The model under review builds one solid part; all positions refer to its coordinate system, in mm. A direction names the side the tool comes from. Round coordinates to 2 decimals unless told otherwise and drop trailing zeros. Order: outer loops, then holes, each group sorted by start corner. A loop starts at its lowest first (then second) coordinate and runs counter-clockwise, first axis right, second up. Notation, with made-up numbers: M -29.5,25 L -12.5,25 A6 cw -12.5,29 Z; hole C 51,88 d11. An arc over 180 degrees is marked long. Answer as a JSON object with one key per item and string values. Group by question number.
1) For faces 1 (the flat face through (-63.5, 1, 0)), 2 (the flat face through (64.146, -12.31, -0.117)), 3 (the cylindrical face through (-41.186, 0.86, -3.874)), list the 3-axis set-ups (+Z, -Z, +X, -X, +Y, -Y) from which the entire face can be reached by the end or side of a thin tool; tool diameter is ignored.
2) Consider section A-A, the plane x = -38. Write out the cut boundary in (y, z), then the cut area to 3 significant figures.
3) The part is to be moulded in two halves that separate along X. For faces 4 (the conical face through (-55.451, 0.681, -3.065)), 5 (the cylindrical face through (-17.218, 0.647, -2.914)), 6 (the cylindrical face through (76.16, -7.92, 10.66)), say which applies: +X half, -X half, draft (parallel to the pull), parting line (faces both ways), or undercut.
4) To check wall thickness, follow line 1 (Z direction, x = -41, y = 0); line 2 (Z direction, x = -27, y = 0); line 3 (X direction, y = -11.5, z = 9.5). State the ranges of each line that lie inside material, in increasing order.
5) Consider section B-B, the plane x = -4. Write out the cut boundary in (y, z).
6) Insertion check: pin 1 Ø4 at (x, z) = (29, -1) entering from -Y; pin 2 Ø6 at (x, z) = (48.5, -5.5) entering from -Y; pin 3 Ø1 at (y, z) = (-16.5, 1.5) entering from +X; pin 4 Ø1.5 at (x, z) = (-26, 5) entering from -Y. Each pin has a flat end and moves straight along its axis. Give the tip position at first contact, or say it passes through.
```python
from build123d import *

# Parameters (mm, degrees)
SWEEP1_PROFILE_R = 2.9845
FILLET1_R        = 2.54


with BuildPart() as part:
    # Sketch1 → Revolve1 (revolve)
    with BuildSketch(Plane.XY):
        Polygon((-63.5, -0.79375), (-63.5, -2.286), (-47.625, -3.96875), (-34.925, -3.96875), (-34.925, -2.9845), (0, -2.9845), (0, -0.79375), align=None)
    revolve(axis=Axis((0, 0, 0), (-1, 0, 0)))

    # Sweep1: sweep along a path in Sketch2
    with BuildLine(Plane.XY) as sweep1_path:
        Line((64.63607564, -8.735441276), (1.72358777, -0.117502426))
        ThreePointArc((1.72358777, -0.117502426), (0.863794191, -0.029409659), (0, 0))
    # Sweep1 profile (on start of the path) → Sweep1 (sweep)
    with BuildSketch(Plane(origin=(64.63607564, -8.735441276, 0), x_dir=(-0.135715572, -0.99074784, 0), z_dir=(-0.99074784, 0.135715572, 0))):
        Circle(SWEEP1_PROFILE_R)
    sweep(path=sweep1_path.line)

    # Sketch15 → Revolve2 (revolve)
    with BuildSketch(Plane.XY):
        Polygon((87.284571273, -11.837899261), (85.802285791, -22.658847175), (63.153790158, -19.556389189), (64.63607564, -8.735441276), align=None)
    revolve(axis=Axis((64.63607564, -8.735441276, 0), (0.99074784, -0.135715572, 0)))

    # Fillet1
    fillet1_edges = [part.edges().sort_by_distance(p)[0] for p in [
        (88.766856755, -1.016951348, 0),
        (66.118361122, 2.085506638, 0),
    ]]
    fillet(fillet1_edges, radius=FILLET1_R)


solid = part.part
```
Results list:
{
 "1": {"face 1": "+Z, -Z, -X, +Y, -Y", "face 2": "none", "face 3": "-X"},
 "2": {"outline": "C 0,0 d7.94; hole C 0,0 d1.59", "area": "47.5 mm^2"},
 "3": {"face 4": "-X half", "face 5": "undercut", "face 6": "parting line"},
 "4": {"line 1": "-3.97 to -0.79, 0.79 to 3.97", "line 2": "-2.98 to -0.79, 0.79 to 2.98", "line 3": "64.75 to 87.07"},
 "5": {"outline": "C 0,0 d5.97; hole C 0,0 d1.59"},
 "6": {"pin 1": "y = -7.11", "pin 2": "y = -8.19", "pin 3": "x = 86.71", "pin 4": "through"}
}
